from build123d import *

# Parameters (mm, degrees)
SKETCH1_W                = 150
SKETCH1_H                = 70
BOSS_EXTRUDE1_DEPTH      = 100
SKETCH2_W                = 40
SKETCH2_H                = 35
CUT_EXTRUDE1_DEPTH       = 100
SKETCH3_W                = 60
SKETCH3_H                = 35
CUT_EXTRUDE2_DEPTH       = 150
BOSS_EXTRUDE2_DEPTH      = 20
BOSS_EXTRUDE2_DEPTH_BACK = 20
SKETCH11_R               = 5
CUT_EXTRUDE4_DEPTH       = 50


with BuildPart() as part:
    # Sketch1 → Boss-Extrude1 (new body)
    with BuildSketch(Plane.XY):
        Rectangle(SKETCH1_W, SKETCH1_H)
    extrude(amount=BOSS_EXTRUDE1_DEPTH)

    # Sketch2 → Cut-Extrude1 (cut)
    with BuildSketch(Plane.XY.offset(100)):
        with Locations((0, -17.5)):
            Rectangle(SKETCH2_W, SKETCH2_H)
    extrude(amount=-CUT_EXTRUDE1_DEPTH, mode=Mode.SUBTRACT)

    # Sketch3 → Cut-Extrude2 (cut)
    with BuildSketch(Plane(origin=(75, 0, 0), x_dir=(0, 0, -1), z_dir=(1, 0, 0))):
        with Locations((-50, -17.5)):
            Rectangle(SKETCH3_W, SKETCH3_H)
    extrude(amount=-CUT_EXTRUDE2_DEPTH, mode=Mode.SUBTRACT)

    # Sketch5 → Boss-Extrude2 (add, two sides: drawn at the far end of the back side and taken through both)
    with BuildSketch(Plane.XY.offset(50).offset(-BOSS_EXTRUDE2_DEPTH_BACK)):
        with BuildLine():
            Line((55, 35), (14.850112855, 104.541644453))
            ThreePointArc((14.850112855, 104.541644453), (-5.074943572, 70.030434377), (-25, 104.541644453))
            Line((-25, 104.541644453), (-55, 104.541644453))
            Line((-55, 104.541644453), (-55, 35))
            Line((-55, 35), (55, 35))
        make_face()
    extrude(amount=BOSS_EXTRUDE2_DEPTH + BOSS_EXTRUDE2_DEPTH_BACK)

    # Sketch11 → Cut-Extrude4 (cut)
    with BuildSketch(Plane(origin=(0, 35, 0), x_dir=(1, 0, 0), z_dir=(0, 1, 0))):
        with Locations(Location((65, -10, 0), (0, 0, 270))):
            Circle(SKETCH11_R)
        with Locations(Location((-65, -10, 0), (0, 0, 270))):
            Circle(SKETCH11_R)
        with Locations(Location((-65, -90, 0), (0, 0, 270))):
            Circle(SKETCH11_R)
        with Locations(Location((65, -90, 0), (0, 0, 270))):
            Circle(SKETCH11_R)
    extrude(amount=-CUT_EXTRUDE4_DEPTH, mode=Mode.SUBTRACT)


solid = part.part
Work out the finished part from the listing and answer in its coordinate system (mm). A direction names the side the tool comes from. Give positions to 0.01 mm unless a question says otherwise; leave off trailing zeros. Loops run counter-clockwise (first coordinate to the right, second up) from the corner with the lowest first, then second, coordinate; pieces in that order, holes last. Notation, with made-up numbers: (75.25, 73) -> (128.25, 73) arc R31 cw to (128.25, 98) -> close; hole circle Ø11 at (13.25, 45.5). An arc over 180 degrees is marked (long way). Use a Markdown table: item, result. Add a question column.
1) Consider line 1 along X through (y, z) = (-2, 90); line 2 along X through (y, z) = (13, 90); line 3 along Z through (x, y) = (-64, 9). Determine where each line is inside the solid, lowest interval first.
2) Each of these flat-tipped pins is pushed along its axis until it touches: P1, Ø21, axis at x = 21, y = 74, coming from the -Z side; P2, Ø10.5, axis at x = -54.5, y = -22.5, coming from the -Z side; P3, Ø10, axis at x = 51.5, z = 47.5, coming from the +Y side; P4, Ø5, axis at x = -65, z = 10, coming from the +Y side. Where does it stop, or does it pass through?
3) The part is cut by section C-C, the plane z = 65. Determine the outline of the cut face in (x, y), plus the area to 3 significant figures.
4) The part is cut by section D-D, the plane x = -65. Determine the outline of the cut face in (y, z), plus the area to 3 significant figures.
5) The part is cut by section B-B, the plane y = 82.5. Determine the outline of the cut face in (x, z).
6) For a pull along X with two mould halves and no side action, classify faces 1 (the flat face through (-65, -15, 90)), 2 (the flat face through (35.21, 69.28, 49.72)), 3 (the flat face through (-75, 7, 49)), 4 (the flat face through (-40, 104.542, 50)) as +X half, -X half, draft (parallel to the pull), parting line (faces both ways), or undercut.
7) Which of the six approach directions +Z, -Z, +X, -X, +Y, -Y give full straight-line access (tool end or side, diameter ignored) to faces 5 (the flat face through (-55, 70, 50)), 6 (the flat face through (-13, 63, 30)), 7 (the flat face through (48, -18, 80)), 8 (the flat face through (65, -15, 90))?
8) The part is cut by section A-A, the plane y = 6. Determine the outline of the cut face in (x, z), plus the area to 3 significant figures.
Reported:
| question | item | result |
|---|---|---|
| 1 | line 1 | x = -75 to -70, -60 to -20, 20 to 60, 70 to 75 |
| 1 | line 2 | x = -75 to -70, -60 to 60, 70 to 75 |
| 1 | line 3 | z = 0 to 5.1, 14.9 to 85.1, 94.9 to 100 |
| 2 | P1 | stops at z = 30 |
| 2 | P2 | stops at z = 0 |
| 2 | P3 | stops at y = 49.72 |
| 2 | P4 | stops at y = -15 |
| 3 | outline | (-75, 0) -> (75, 0) -> (75, 35) -> (55, 35) -> (14.85, 104.54) arc R23.01 cw (long way) to (-25, 104.54) -> (-55, 104.54) -> (-55, 35) -> (-75, 35) -> close |
| 3 | area | 10,200 mm^2 |
| 4 | outline | (-35, 0) -> (35, 0) -> (35, 5) -> (-15, 5) -> (-15, 15) -> (35, 15) -> (35, 85) -> (-15, 85) -> (-15, 95) -> (35, 95) -> (35, 100) -> (-35, 100) -> (-35, 80) -> (0, 80) -> (0, 20) -> (-35, 20) -> close |
| 4 | area | 3,900 mm^2 |
| 5 | outline | (-55, 30) -> (-25.53, 30) -> (-25.53, 70) -> (-55, 70) -> close; (15.38, 30) -> (27.58, 30) -> (27.58, 70) -> (15.38, 70) -> close |
| 6 | face 1 | undercut |
| 6 | face 2 | +X half |
| 6 | face 3 | -X half |
| 6 | face 4 | draft |
| 7 | face 5 | +Z, -Z, -X, +Y |
| 7 | face 6 | -Z, +X, -X, +Y |
| 7 | face 7 | +X, -X, -Y |
| 7 | face 8 | +Y |
| 8 | outline | (-75, 0) -> (75, 0) -> (75, 100) -> (-75, 100) -> close; hole circle Ø10 at (-65, 10); hole circle Ø10 at (-65, 90); hole circle Ø10 at (65, 10); hole circle Ø10 at (65, 90) |
| 8 | area | 14,700 mm^2 |
